from build123d import *

# Parameters (mm, degrees)
SKETCH1_W                                     = 940.88204
SKETCH1_H                                     = 454.025
SKETCH1_R                                     = 3.3734375
BOSS_EXTRUDE1_DEPTH                           = 12.7
FILLET1_R                                     = 3.175
SKETCH2_W                                     = 269.875
SKETCH2_H                                     = 269.875
CUT_EXTRUDE1_DEPTH                            = 7.9375
FILLET2_R                                     = 3.175
CSK_FOR_1_4_FLAT_HEAD_MACHINE_SCREW1_AT_COUNT = 2
CSK_FOR_1_4_FLAT_HEAD_MACHINE_SCREW1_AT_PITCH = 763.08204
CSK_FOR_1_4_FLAT_HEAD_MACHINE_SCREW1_2_COUNT  = 2
CSK_FOR_1_4_FLAT_HEAD_MACHINE_SCREW1_2_PITCH  = 330.2
CSK_FOR_1_4_FLAT_HEAD_MACHINE_SCREW1_3_COUNT  = 2
CSK_FOR_1_4_FLAT_HEAD_MACHINE_SCREW1_3_PITCH  = 422.803622168
CSK_FOR_1_4_FLAT_HEAD_MACHINE_SCREW1_4_COUNT  = 2
CSK_FOR_1_4_FLAT_HEAD_MACHINE_SCREW1_4_PITCH  = 598.371981477
CSK_FOR_1_4_FLAT_HEAD_MACHINE_SCREW1_5_COUNT  = 2
CSK_FOR_1_4_FLAT_HEAD_MACHINE_SCREW1_5_PITCH  = 831.460305589


with BuildPart() as part:
    # Sketch1 → Boss-Extrude1 (new body)
    with BuildSketch(Plane(origin=(0, 0, 0), x_dir=(0, 0, -1), z_dir=(1, 0, 0))):
        with Locations((470.44102, 227.0125)):
            Rectangle(SKETCH1_W, SKETCH1_H)
        with Locations((352.96602, 422.275)):
            Circle(SKETCH1_R, mode=Mode.SUBTRACT)
        with Locations((587.91602, 422.275)):
            Circle(SKETCH1_R, mode=Mode.SUBTRACT)
    extrude(amount=BOSS_EXTRUDE1_DEPTH)

    # Fillet1
    fillet1_edges = [part.edges().sort_by_distance(p)[0] for p in [
        (6.35, 454.025, 0),
        (6.35, 454.025, -940.88204),
        (6.35, 0, -940.88204),
        (6.35, 0, 0),
    ]]
    fillet(fillet1_edges, radius=FILLET1_R)

    # Sketch2 → Cut-Extrude1 (cut)
    with BuildSketch(Plane(origin=(12.7, 0, 0), x_dir=(0, 0, -1), z_dir=(1, 0, 0))):
        with Locations((470.44102, 304.8)):
            Rectangle(SKETCH2_W, SKETCH2_H)
    extrude(amount=-CUT_EXTRUDE1_DEPTH, mode=Mode.SUBTRACT)

    # Fillet2
    fillet2_edges = [part.edges().sort_by_distance(p)[0] for p in [
        (8.73125, 169.8625, -335.50352),
        (8.73125, 439.7375, -335.50352),
        (8.73125, 439.7375, -605.37852),
        (8.73125, 169.8625, -605.37852),
    ]]
    fillet(fillet2_edges, radius=FILLET2_R)

    # Sketch5 → CSK for 1/4 Flat Head Machine Screw1 (revolve, cut)
    with BuildSketch(Plane(origin=(12.7, 374.65, -88.9), x_dir=(0, 0, -1), z_dir=(0, 1, 0))):
        Polygon((0, 0), (0, 12.7), (3.3782, 12.7), (3.3782, 4.536932584), (6.4389, 1.016), (6.4389, 0), align=None)
    csk_for_1_4_flat_head_machine_screw1 = revolve(axis=Axis((19.05, 374.65, -88.9), (-1, 0, 0)), mode=Mode.SUBTRACT)

    # CSK for 1/4 Flat Head Machine Screw1 at: CSK for 1/4 Flat Head Machine Screw1 ×2
    with Locations(*[(0, 0, -i * CSK_FOR_1_4_FLAT_HEAD_MACHINE_SCREW1_AT_PITCH) for i in range(1, CSK_FOR_1_4_FLAT_HEAD_MACHINE_SCREW1_AT_COUNT)]):
        add(csk_for_1_4_flat_head_machine_screw1, mode=Mode.SUBTRACT)

    # CSK for 1_4 Flat Head Machine Screw1 2: CSK for 1/4 Flat Head Machine Screw1 ×2
    with Locations(*[(0, -i * CSK_FOR_1_4_FLAT_HEAD_MACHINE_SCREW1_2_PITCH, 0) for i in range(1, CSK_FOR_1_4_FLAT_HEAD_MACHINE_SCREW1_2_COUNT)]):
        add(csk_for_1_4_flat_head_machine_screw1, mode=Mode.SUBTRACT)

    # CSK for 1_4 Flat Head Machine Screw1 3: CSK for 1/4 Flat Head Machine Screw1 ×2
    with Locations(*[Vector(0, -0.780977226, -0.624559503) * (i * CSK_FOR_1_4_FLAT_HEAD_MACHINE_SCREW1_3_PITCH) for i in range(1, CSK_FOR_1_4_FLAT_HEAD_MACHINE_SCREW1_3_COUNT)]):
        add(csk_for_1_4_flat_head_machine_screw1, mode=Mode.SUBTRACT)

    # CSK for 1_4 Flat Head Machine Screw1 4: CSK for 1/4 Flat Head Machine Screw1 ×2
    with Locations(*[Vector(0, -0.551830651, -0.833956194) * (i * CSK_FOR_1_4_FLAT_HEAD_MACHINE_SCREW1_4_PITCH) for i in range(1, CSK_FOR_1_4_FLAT_HEAD_MACHINE_SCREW1_4_COUNT)]):
        add(csk_for_1_4_flat_head_machine_screw1, mode=Mode.SUBTRACT)

    # CSK for 1_4 Flat Head Machine Screw1 5: CSK for 1/4 Flat Head Machine Screw1 ×2
    with Locations(*[Vector(0, -0.397132608, -0.917761239) * (i * CSK_FOR_1_4_FLAT_HEAD_MACHINE_SCREW1_5_PITCH) for i in range(1, CSK_FOR_1_4_FLAT_HEAD_MACHINE_SCREW1_5_COUNT)]):
        add(csk_for_1_4_flat_head_machine_screw1, mode=Mode.SUBTRACT)


solid = part.part
For this review, take the finished solid that the model builds, in its own axes (mm). Round coordinates to 2 decimals unless told otherwise and drop trailing zeros. Order: outer loops, then holes, each group sorted by start corner. A loop starts at its lowest first (then second) coordinate and runs counter-clockwise, first axis right, second up. Notation, with made-up numbers: (16, 72.5) -> (52, 72.5) arc R30 cw to (52, 107.5) -> close; hole circle Ø6 at (46, 30). An arc over 180 degrees is marked (long way). Write item = value, one per line. Start each with the question number.
1) Insertion check: pin 1 (11 mm diameter, centred on y = 374.65, z = -88.9, fed in from +X); pin 2 (20.5 mm diameter, centred on y = 374.65, z = -88.9, fed in from +X); pin 3 (8 mm diameter, centred on y = 44.45, z = -352.97, fed in from +X); pin 4 (5.5 mm diameter, centred on y = 374.65, z = -851.98, fed in from -X). Each pin has a flat end and moves straight along its axis. Give the tip position at first contact, or say it passes through.
2) To check wall thickness, follow line 1 (Z direction, x = 2.25, y = 374.65); line 2 (Z direction, x = 6.75, y = 231); line 3 (Z direction, x = 12.05, y = 374.65). State the ranges of each line that lie inside material, in increasing order. Write a range as from..to.
3) Take a section at A-A on y = 223. State the section outline as (x, z) points, plus the area to 3 significant figures.
4) Take a section at B-B on z = -442. State the section outline as (x, y) points (1 decimal).
5) The part is to be moulded in two halves that separate along Y. For faces 1 (the face through (12.7, 129, -464)), 2 (the face through (4.762, 307, -469)), say which applies: +Y half, -Y half, draft (parallel to the pull), parting line (faces both ways), or undercut.
Verdict:
q1.pin_1 = 10.6
q1.pin_2 = 12.7
q1.pin_3 = 8.88
q1.pin_4 = through
q2.line_1 = -940.88..-855.36, -848.6..-92.28, -85.52..0
q2.line_2 = -940.88..-605.38, -335.5..0
q2.line_3 = -940.88..-858.42, -845.54..-605.38, -335.5..-95.34, -82.46..0
q3.outline = (0, -940.88) -> (12.7, -940.88) -> (12.7, -605.38) -> (4.76, -605.38) -> (4.76, -335.5) -> (12.7, -335.5) -> (12.7, 0) -> (0, 0) -> close
q3.area = 9,810 mm2
q4.outline = (0, 0) -> (12.7, 0) -> (12.7, 169.9) -> (4.8, 169.9) -> (4.8, 439.7) -> (12.7, 439.7) -> (12.7, 454) -> (0, 454) -> close
q5.face_1 = draft
q5.face_2 = undercut
